```python
from build123d import *

# Parameters (mm, degrees)
SKETCH1_W           = 60
SKETCH1_H           = 50
BOSS_EXTRUDE1_DEPTH = 3
SKETCH2_W           = 9
SKETCH2_H           = 17
BOSS_EXTRUDE2_DEPTH = 160
SKETCH3_W           = 4.5
SKETCH3_H           = 3
CUT_EXTRUDE1_DEPTH  = 157
CUT_EXTRUDE2_START  = 26
SKETCH4_R           = 1.45
CUT_EXTRUDE2_DEPTH  = 5
CUT_EXTRUDE3_REACH  = 166.697
SKETCH5_R           = 2
SKETCH8_W           = 30
SKETCH8_H           = 10
BOSS_EXTRUDE3_DEPTH = 0.0001
CUT_EXTRUDE4_REACH  = 166.697
SKETCH9_R           = 1.863373193


with BuildPart() as part:
    # Sketch1 → Boss-Extrude1 (new body)
    with BuildSketch(Plane(origin=(0, 0, 0), x_dir=(1, 0, 0), z_dir=(0, 1, 0))):
        Rectangle(SKETCH1_W, SKETCH1_H)
    extrude(amount=BOSS_EXTRUDE1_DEPTH)

    # Sketch2 → Boss-Extrude2 (add)
    with BuildSketch(Plane(origin=(0, 3, 0), x_dir=(1, 0, 0), z_dir=(0, 1, 0))):
        with Locations((17.5, 0)):
            Rectangle(SKETCH2_W, SKETCH2_H)
        with Locations((-17.5, 0)):
            Rectangle(SKETCH2_W, SKETCH2_H)
    extrude(amount=BOSS_EXTRUDE2_DEPTH)

    # Sketch3 → Cut-Extrude1 (cut)
    with BuildSketch(Plane(origin=(0, 163, 0), x_dir=(1, 0, 0), z_dir=(0, 1, 0))):
        with Locations((-15.25, 4)):
            Rectangle(SKETCH3_W, SKETCH3_H)
        with Locations((-15.25, -4)):
            Rectangle(SKETCH3_W, SKETCH3_H)
        with Locations((15.25, -4)):
            Rectangle(SKETCH3_W, SKETCH3_H)
        with Locations((15.25, 4)):
            Rectangle(SKETCH3_W, SKETCH3_H)
    extrude(amount=-CUT_EXTRUDE1_DEPTH, mode=Mode.SUBTRACT)

    # Sketch4 → Cut-Extrude2 (cut)
    with BuildSketch(Plane(origin=(-13, 0, 0), x_dir=(0, 0, -1), z_dir=(1, 0, 0)).offset(CUT_EXTRUDE2_START)):
        with Locations((0, 7)):
            Circle(SKETCH4_R)
        with Locations((0, 160)):
            Circle(SKETCH4_R)
    extrude(amount=CUT_EXTRUDE2_DEPTH, mode=Mode.SUBTRACT)

    # Sketch5 → Cut-Extrude3 (cut, up to next)
    with BuildSketch(Plane(origin=(0, 3, 0), x_dir=(1, 0, 0), z_dir=(0, 1, 0)), mode=Mode.PRIVATE) as cut_extrude3_sk1:
        with Locations(Location((-24, 14, 0), (0, 0, 270))):
            Circle(SKETCH5_R)
    cut_extrude3_tool1 = extrude(cut_extrude3_sk1.sketch, amount=-CUT_EXTRUDE3_REACH, mode=Mode.PRIVATE) & part.part
    # Sketch5 → Cut-Extrude3 (cut, up to next)
    with BuildSketch(Plane(origin=(0, 3, 0), x_dir=(1, 0, 0), z_dir=(0, 1, 0)), mode=Mode.PRIVATE) as cut_extrude3_sk2:
        with Locations(Location((-24, -14, 0), (0, 0, 270))):
            Circle(SKETCH5_R)
    cut_extrude3_tool2 = extrude(cut_extrude3_sk2.sketch, amount=-CUT_EXTRUDE3_REACH, mode=Mode.PRIVATE) & part.part
    # Sketch5 → Cut-Extrude3 (cut, up to next)
    with BuildSketch(Plane(origin=(0, 3, 0), x_dir=(1, 0, 0), z_dir=(0, 1, 0)), mode=Mode.PRIVATE) as cut_extrude3_sk3:
        with Locations(Location((24, -14, 0), (0, 0, 270))):
            Circle(SKETCH5_R)
    cut_extrude3_tool3 = extrude(cut_extrude3_sk3.sketch, amount=-CUT_EXTRUDE3_REACH, mode=Mode.PRIVATE) & part.part
    # Sketch5 → Cut-Extrude3 (cut, up to next)
    with BuildSketch(Plane(origin=(0, 3, 0), x_dir=(1, 0, 0), z_dir=(0, 1, 0)), mode=Mode.PRIVATE) as cut_extrude3_sk4:
        with Locations(Location((24, 14, 0), (0, 0, 270))):
            Circle(SKETCH5_R)
    cut_extrude3_tool4 = extrude(cut_extrude3_sk4.sketch, amount=-CUT_EXTRUDE3_REACH, mode=Mode.PRIVATE) & part.part
    add(cut_extrude3_tool1.solids().sort_by_distance((-24, 3, -14))[0], mode=Mode.SUBTRACT)
    add(cut_extrude3_tool2.solids().sort_by_distance((-24, 3, 14))[0], mode=Mode.SUBTRACT)
    add(cut_extrude3_tool3.solids().sort_by_distance((24, 3, 14))[0], mode=Mode.SUBTRACT)
    add(cut_extrude3_tool4.solids().sort_by_distance((24, 3, -14))[0], mode=Mode.SUBTRACT)

    # Sketch8 → Boss-Extrude3 (add)
    with BuildSketch(Plane(origin=(0, 3, 0), x_dir=(1, 0, 0), z_dir=(0, 1, 0))):
        with Locations((0, 20)):
            Rectangle(SKETCH8_W, SKETCH8_H)
    extrude(amount=BOSS_EXTRUDE3_DEPTH)

    # Sketch9 → Cut-Extrude4 (cut, up to next)
    with BuildSketch(Plane(origin=(0, 3.0001, 0), x_dir=(1, 0, 0), z_dir=(0, 1, 0)), mode=Mode.PRIVATE) as cut_extrude4_sk1:
        with Locations(Location((-9, 20, 0), (0, 0, 270))):
            Circle(SKETCH9_R)
    cut_extrude4_tool1 = extrude(cut_extrude4_sk1.sketch, amount=-CUT_EXTRUDE4_REACH, mode=Mode.PRIVATE) & part.part
    # Sketch9 → Cut-Extrude4 (cut, up to next)
    with BuildSketch(Plane(origin=(0, 3.0001, 0), x_dir=(1, 0, 0), z_dir=(0, 1, 0)), mode=Mode.PRIVATE) as cut_extrude4_sk2:
        with Locations(Location((9, 20, 0), (0, 0, 270))):
            Circle(SKETCH9_R)
    cut_extrude4_tool2 = extrude(cut_extrude4_sk2.sketch, amount=-CUT_EXTRUDE4_REACH, mode=Mode.PRIVATE) & part.part
    add(cut_extrude4_tool1.solids().sort_by_distance((-9, 3.0001, -20))[0], mode=Mode.SUBTRACT)
    add(cut_extrude4_tool2.solids().sort_by_distance((9, 3.0001, -20))[0], mode=Mode.SUBTRACT)


solid = part.part
```
Input: part model. Units: mm. Frame: model coordinates. A direction names the side the tool comes from. Coordinates: 2 decimals unless noted, no trailing zeros. Write each loop counter-clockwise with the first axis right and the second up, starting at its lowest first coordinate (ties: lowest second). Pieces come first, ordered by that corner, then holes. Notation, with made-up numbers: (-13, -5.5) - (14, -5.5) arc R26 ccw to (14, 17.5) - close; hole circle Ø11 at (3, 52). An arc over 180 degrees is marked (long way). Put each result on its own line as item: value. Start each with the question number.
1) Reachability of faces 1 (the face through (15.465, 158.584, 0.314)), 2 (the face through (17, 82, -8.5)), 3 (the face through (15, 86, 2.5)) from +Z, -Z, +X, -X, +Y, -Y: full face, straight path, thin tool, end or side. Return the list, or none.
2) Cut plane A-A (z = -20). State how many separate pieces and enclosed holes the cut face has, plus the area to 3 significant figures.
3) Mould query, pull axis Z, two halves, no side actions, for faces 4 (the face through (-18, 82, 8.5)), 5 (the face through (18, 7, 0)), 6 (the face through (-30, 1, 0)), 7 (the face through (17.5, 86, -4)). Classes: pulls with the +Z half, pulls with the -Z half, needs draft (parallel to the pull), parting line crosses it, or undercut.
4) Ray query, L1, parallel to X at y = 2, z = 14; L2, parallel to X at y = 1.65, z = -20; L3, parallel to Y at x = 16, z = 0. Return the intervals inside material, ascending.
5) Cut plane C-C (y = 160). Return the cut outline in (x, z), plus the area to 4 significant figures.
6) Cut plane B-B (y = 94). Return the cut outline in (x, z).
7) Contact query for flat-ended pins moving along their axis: pin 1 (5 mm diameter, centred on x = 24, z = -14, fed in from -Y); pin 2 (5 mm diameter, centred on x = 16, y = 56, fed in from +Z); pin 3 (8 mm diameter, centred on x = -1, z = -19.5, fed in from +Y); pin 4 (3 mm diameter, centred on y = 79.5, z = 3.5, fed in from +X). Output: stop coordinate, or through.
Resolved:
1. face 1: none
1. face 2: -Z, +X, -X, +Y
1. face 3: +Y
2. separate pieces: 3
2. enclosed holes: 0
2. area: 158 mm2
3. face 4: pulls with the +Z half
3. face 5: undercut
3. face 6: needs draft
3. face 7: undercut
4. L1: x = -30 to -26, -22 to 22, 26 to 30
4. L2: x = -30 to -10.86, -7.14 to 7.14, 10.86 to 30
4. L3: y = 0 to 5.55, 8.45 to 158.55, 161.45 to 163
5. outline: (-22, -8.5) - (-13, -8.5) - (-13, -5.5) - (-17.5, -5.5) - (-17.5, -2.5) - (-13, -2.5) - (-13, 2.5) - (-17.5, 2.5) - (-17.5, 5.5) - (-13, 5.5) - (-13, 8.5) - (-22, 8.5) - close; (13, -8.5) - (22, -8.5) - (22, 8.5) - (13, 8.5) - (13, 5.5) - (17.5, 5.5) - (17.5, 2.5) - (13, 2.5) - (13, 1.45) - (18, 1.45) - (18, -1.45) - (13, -1.45) - (13, -2.5) - (17.5, -2.5) - (17.5, -5.5) - (13, -5.5) - close
5. area: 237.5 mm2
6. outline: (-22, -8.5) - (-13, -8.5) - (-13, -5.5) - (-17.5, -5.5) - (-17.5, -2.5) - (-13, -2.5) - (-13, 2.5) - (-17.5, 2.5) - (-17.5, 5.5) - (-13, 5.5) - (-13, 8.5) - (-22, 8.5) - close; (13, -8.5) - (22, -8.5) - (22, 8.5) - (13, 8.5) - (13, 5.5) - (17.5, 5.5) - (17.5, 2.5) - (13, 2.5) - (13, -2.5) - (17.5, -2.5) - (17.5, -5.5) - (13, -5.5) - close
7. pin 1: stops at y = 0
7. pin 2: stops at z = 8.5
7. pin 3: stops at y = 3
7. pin 4: stops at x = 22
